from build123d import *

# Parameters (mm, degrees)
SKIZZE2_R                       = 21.35
AUFSATZ_LINEAR_AUSTRAGEN1_DEPTH = 2
SKIZZE6_R                       = 10.05
SCHNITT_LINEAR_AUSTRAGEN4_DEPTH = 31.259626567
SKIZZE7_R                       = 16
SCHNITT_LINEAR_AUSTRAGEN5_DEPTH = 0.6
FASE1_SIZE                      = 1.1
FASE1_SIZE2                     = 6.238410002
SKIZZE8_R                       = 12.65
SCHNITT_LINEAR_AUSTRAGEN6_DEPTH = 0.1


with BuildPart() as part:
    # Skizze2 → Aufsatz-Linear austragen1 (new body)
    with BuildSketch(Plane.XY):
        Circle(SKIZZE2_R)
    extrude(amount=AUFSATZ_LINEAR_AUSTRAGEN1_DEPTH)

    # Skizze6 → Schnitt-Linear austragen4 (cut, through all)
    with BuildSketch(Plane.XY.offset(2)):
        Circle(SKIZZE6_R)
    extrude(amount=-SCHNITT_LINEAR_AUSTRAGEN4_DEPTH, mode=Mode.SUBTRACT)

    # Skizze7 → Schnitt-Linear austragen5 (cut)
    with BuildSketch(Plane.XY.offset(2)):
        Circle(SKIZZE7_R)
    extrude(amount=-SCHNITT_LINEAR_AUSTRAGEN5_DEPTH, mode=Mode.SUBTRACT)

    # Fase1
    fase1_edges = [part.edges().sort_by_distance(p)[0] for p in [
        (-10.05, 0, 0),
    ]]
    fase1_side = [part.faces().sort_by_distance(p)[0] for p in [
        (-10.05, 0, 0.7),
    ]]
    chamfer(fase1_edges, length=FASE1_SIZE, length2=FASE1_SIZE2, reference=fase1_side[0])

    # Skizze8 → Schnitt-Linear austragen6 (cut)
    with BuildSketch(Plane.XY.offset(1.4)):
        Circle(SKIZZE8_R)
    extrude(amount=-SCHNITT_LINEAR_AUSTRAGEN6_DEPTH, mode=Mode.SUBTRACT)


solid = part.part
Geometry check sheet. Reference: the model listing, model coordinates, mm. A direction names the side the tool comes from. Give positions to 0.01 mm unless a question says otherwise; leave off trailing zeros. Write each loop counter-clockwise with the first axis right and the second up, starting at its lowest first coordinate (ties: lowest second). Pieces come first, ordered by that corner, then holes. Notation, with made-up numbers: M 24.5,12.25 L 35.5,12.25 A21 cw 35.5,18.25 Z; hole C 26,-10 d3. An arc over 180 degrees is marked long. Answer as CSV lines item,"result". Start each with the question number.
Q1. Release check for a two-part mould opening along X. For faces 1 (the face through (-3.47, -15.62, 1.7)), 2 (the face through (-4.63, -20.84, 0.99)), 3 (the face through (-5, -16, 0)), 4 (the face through (-2.26, -10.19, 1.03)) record: pulls with the +X half, pulls with the -X half, needs draft (parallel to the pull), parting line crosses it, or undercut.
Q2. Material ranges on L1, parallel to Y at x = 0, z = 1.45; L2, parallel to Y at x = 0, z = 1.25; L3, parallel to Z at x = 11, y = -12, recorded low to high.
Q3. Go/stop test with flat-tipped pins: pin 1 (5 mm diameter, centred on x = -8.5, y = 1.5, fed in from +Z); pin 2 (19 mm diameter, centred on x = 0, y = 0, fed in from -Z); pin 3 (5 mm diameter, centred on x = 11, y = 0, fed in from +Z); pin 4 (12 mm diameter, centred on x = 8.5, y = -8.5, fed in from +Z). Record where each tip stops, or that it passes through.
Q4. Section check A-A, the plane y = 0. Record the cut outline in (x, z).
Q5. Section check D-D, the plane x = 18.5. Record the cut outline in (y, z), then the cut area to 3 significant figures.
Q6. Section check C-C, the plane z = 0.45. Record the cut outline in (x, y), then the cut area to 3 significant figures.
Q7. Tool access check on faces 5 (the face through (3, 16, 2)), 6 (the face through (0.9, 10.4, 1.3)). Record the directions out of +Z, -Z, +X, -X, +Y, -Y that give a thin tool (end or side, any length) a straight path to the whole face; none if there is none.
Geometry says:
1,face 1,"undercut"
1,face 2,"parting line crosses it"
1,face 3,"needs draft"
1,face 4,"undercut"
2,L1,"-21.35 to -16, 16 to 21.35"
2,L2,"-21.35 to -10.05, 10.05 to 21.35"
2,L3,"0 to 2"
3,pin 1,"z = 1.3"
3,pin 2,"through"
3,pin 3,"z = 1.4"
3,pin 4,"z = 2"
4,outline,"M -21.35,0 L -16.29,0 L -10.05,1.1 L -10.05,1.3 L -12.65,1.3 L -12.65,1.4 L -16,1.4 L -16,2 L -21.35,2 Z; M 10.05,1.1 L 16.29,0 L 21.35,0 L 21.35,2 L 16,2 L 16,1.4 L 12.65,1.4 L 12.65,1.3 L 10.05,1.3 Z"
5,outline,"M -10.66,0 L 10.66,0 L 10.66,2 L -10.66,2 Z"
5,area,"42.6 mm^2"
6,outline,"C 0,0 d42.7; hole C 0,0 d27.47"
6,area,"839 mm^2"
7,face 5,"+Z, +X, -X, +Y, -Y"
7,face 6,"+Z"
